Work out the finished part from the listing and answer in its coordinate system (mm). A direction names the side the tool comes from. Coordinates: 2 decimals unless noted, no trailing zeros. Write each loop counter-clockwise with the first axis right and the second up, starting at its lowest first coordinate (ties: lowest second). Pieces come first, ordered by that corner, then holes. Notation, with made-up numbers: (65.25, 5) - (79.25, 5) arc R31 cw to (79.25, 34) - close; hole circle Ø8 at (88, 70). An arc over 180 degrees is marked (long way). Use one line per item in the form item = value. Start each with the question number.
Item 1: A cutting plane is placed at B-B (z = 2). Write down the section's boundary in (x, y), then the cut area to 3 significant figures.
Item 2: Determine the mould class of faces 6 (the flat face through (-8.5, 5.3, 0.8)), 7 (the flat face through (-10, -11, 1)), 8 (the cylindrical face through (-8.63, -7.51, 0.79)) for opening direction Y: released by +Y, released by -Y, zero draft, split by the parting line, or undercut.
Item 3: Given pin 1 (0.9 mm diameter, centred on y = 0, z = 2.5, fed in from +X); pin 2 (1 mm diameter, centred on x = -8.5, y = -2, fed in from +Z); pin 3 (2 mm diameter, centred on y = -0.5, z = 3, fed in from +X), each flat-ended and moving along its own axis, determine where each tip first touches the part or whether it passes through.
Item 4: Consider probe 1 along X at (y, z) = (-6, 1.25); probe 2 along Y at (x, z) = (-2.54, 0.35); probe 3 along Z at (x, y) = (8.5, 0.5). Determine where each line is inside the solid, lowest interval first.
Item 5: For faces 1 (the flat face through (11.5, -2, 1)), 2 (the flat face through (0, -9, 1.6)), 3 (the flat face through (-5, -2, 2.61)), 4 (the cylindrical face through (-0.052, -6.103, 0.799)), 5 (the flat face through (3.5, -2, 2)), determine the directions among +Z, -Z, +X, -X, +Y, -Y from which every point of the face is accessible in a straight line to the end or side of a thin tool.
from build123d import *

# Parameters (mm, degrees)
SKETCH1_R           = 1
BOSS_EXTRUDE1_DEPTH = 1.6
SKETCH2_W           = 17
SKETCH2_H           = 12
BOSS_EXTRUDE2_DEPTH = 1.61
SKETCH3_W           = 14
SKETCH3_H           = 2.4
SKETCH3_W_2         = 13.6
SKETCH3_H_2         = 2
SKETCH3_R           = 0.6
SKETCH3_R_2         = 0.4
BOSS_EXTRUDE3_DEPTH = 1.62
SKETCH3_3_R         = 0.4
CUT_EXTRUDE1_DEPTH  = 2.62
BOSS_EXTRUDE4_START = 1.61
SKETCH4_W           = 3.8
SKETCH4_H           = 5
BOSS_EXTRUDE4_DEPTH = 2
BOSS_EXTRUDE5_START = 1.61
SKETCH5_W           = 2
SKETCH5_H           = 1.2
BOSS_EXTRUDE5_DEPTH = 1
CHAMFER1_SIZE       = 0.3
SKETCH6_R           = 1
SKETCH6_W           = 23
SKETCH6_H           = 6
CUT_EXTRUDE2_DEPTH  = 2


with BuildPart() as part:
    # Sketch1 → Boss-Extrude1 (new body)
    with BuildSketch(Plane.XY):
        Polygon((-11.5, 9.5), (-9.5, 11.5), (9.5, 11.5), (11.5, 9.5), (11.5, -9.5), (9.5, -11.5), (-9.5, -11.5), (-11.5, -9.5), align=None)
        with Locations((-9, 6)):
            Circle(SKETCH1_R, mode=Mode.SUBTRACT)
        with Locations((9, 6)):
            Circle(SKETCH1_R, mode=Mode.SUBTRACT)
        with Locations((-9, -6)):
            Circle(SKETCH1_R, mode=Mode.SUBTRACT)
        with Locations((9, -6)):
            Circle(SKETCH1_R, mode=Mode.SUBTRACT)
        with Locations((8.5, -8.5)):
            Circle(SKETCH1_R, mode=Mode.SUBTRACT)
        with Locations((-8.5, -8.5)):
            Circle(SKETCH1_R, mode=Mode.SUBTRACT)
    extrude(amount=BOSS_EXTRUDE1_DEPTH)

    # Sketch2 → Boss-Extrude2 (add)
    with BuildSketch(Plane.XY):
        Rectangle(SKETCH2_W, SKETCH2_H)
    extrude(amount=BOSS_EXTRUDE2_DEPTH)

    # Sketch3 → Boss-Extrude3 (add)
    with BuildSketch(Plane.XY):
        with Locations((0, -6.5)):
            Rectangle(SKETCH3_W, SKETCH3_H)
        with Locations((0, -6.5)):
            Rectangle(SKETCH3_W_2, SKETCH3_H_2, mode=Mode.SUBTRACT)
        with Locations(Location((-5.08, -6.5, 0), (0, 0, 123.557309762))):
            Circle(SKETCH3_R)
        with Locations((-5.08, -6.5)):
            Circle(SKETCH3_R_2, mode=Mode.SUBTRACT)
        with Locations(Location((-2.54, -6.5, 0), (0, 0, 123.557309762))):
            Circle(SKETCH3_R)
        with Locations((-2.54, -6.5)):
            Circle(SKETCH3_R_2, mode=Mode.SUBTRACT)
        with Locations(Location((0, -6.5, 0), (0, 0, 123.557309762))):
            Circle(SKETCH3_R)
        with Locations((0, -6.5)):
            Circle(SKETCH3_R_2, mode=Mode.SUBTRACT)
        with Locations(Location((5.08, -6.5, 0), (0, 0, 123.557309762))):
            Circle(SKETCH3_R)
        with Locations((5.08, -6.5)):
            Circle(SKETCH3_R_2, mode=Mode.SUBTRACT)
        with Locations(Location((2.54, -6.5, 0), (0, 0, 123.557309762))):
            Circle(SKETCH3_R)
        with Locations((2.54, -6.5)):
            Circle(SKETCH3_R_2, mode=Mode.SUBTRACT)
    extrude(amount=BOSS_EXTRUDE3_DEPTH)

    # Sketch3<3> → Cut-Extrude1 (cut)
    with BuildSketch(Plane.XY):
        with Locations((-5.08, -6.5)):
            Circle(SKETCH3_3_R)
        with Locations((-2.54, -6.5)):
            Circle(SKETCH3_3_R)
        with Locations((0, -6.5)):
            Circle(SKETCH3_3_R)
        with Locations((2.54, -6.5)):
            Circle(SKETCH3_3_R)
        with Locations((5.08, -6.5)):
            Circle(SKETCH3_3_R)
    extrude(amount=CUT_EXTRUDE1_DEPTH, mode=Mode.SUBTRACT)

    # Sketch4 → Boss-Extrude4 (add)
    with BuildSketch(Plane.XY.offset(BOSS_EXTRUDE4_START)):
        Rectangle(SKETCH4_W, SKETCH4_H)
    extrude(amount=BOSS_EXTRUDE4_DEPTH)

    # Sketch5 → Boss-Extrude5 (add)
    with BuildSketch(Plane.XY.offset(BOSS_EXTRUDE5_START)):
        with Locations((-4.500129294, -1.9)):
            Rectangle(SKETCH5_W, SKETCH5_H)
        with Locations((-4.5, 0.5)):
            Rectangle(SKETCH5_W, SKETCH5_H)
        with Locations((4.5, -1.9)):
            Rectangle(SKETCH5_W, SKETCH5_H)
    extrude(amount=BOSS_EXTRUDE5_DEPTH)

    # Chamfer1
    chamfer1_edges = [part.edges().sort_by_distance(p)[0] for p in [
        (1.9, 0, 3.61),
        (0, 2.5, 3.61),
        (-1.9, 0, 3.61),
        (0, -2.5, 3.61),
    ]]
    chamfer(chamfer1_edges, length=CHAMFER1_SIZE)

    # Sketch6 → Cut-Extrude2 (cut)
    with BuildSketch(Plane.XY):
        with Locations(Location((9, -6, 0), (0, 0, 180))):
            Circle(SKETCH6_R)
        with Locations((-9, -6)):
            Circle(SKETCH6_R)
        with Locations((0, 8.5)):
            Rectangle(SKETCH6_W, SKETCH6_H)
    extrude(amount=CUT_EXTRUDE2_DEPTH, mode=Mode.SUBTRACT)


solid = part.part
Answer:
q1.outline = (-5.5, -2.5) - (-3.5, -2.5) - (-3.5, -1.3) - (-5.5, -1.3) - close; (-5.5, -0.1) - (-3.5, -0.1) - (-3.5, 1.1) - (-5.5, 1.1) - close; (-1.9, -2.5) - (1.9, -2.5) - (1.9, 2.5) - (-1.9, 2.5) - close; (3.5, -2.5) - (5.5, -2.5) - (5.5, -1.3) - (3.5, -1.3) - close
q1.area = 26.2 mm²
q2.face_6 = zero draft
q2.face_7 = released by -Y
q2.face_8 = undercut
q3.pin_1 = 1.9
q3.pin_2 = 1.61
q3.pin_3 = 5.5
q4.probe_1 = -11.5 to -10, -8 to 8, 10 to 11.5
q4.probe_2 = -11.5 to -6.9, -6.1 to 5.5
q4.probe_3 = 0 to 1.6
q5.face_1 = +Z, -Z, +X, +Y, -Y
q5.face_2 = +Z, -Y
q5.face_3 = +Z, -X, +Y, -Y
q5.face_4 = +Z, -Z
q5.face_5 = +Z, +Y, -Y
